Can you work these out from the model? Positions are in its coordinate system, mm. A direction names the side the tool comes from. Give positions to 0.01 mm unless a question says otherwise; leave off trailing zeros. Order: outer loops, then holes, each group sorted by start corner. A loop starts at its lowest first (then second) coordinate and runs counter-clockwise, first axis right, second up. Notation, with made-up numbers: M -7,11.5 L 2,11.5 A22 cw 2,23.5 Z; hole C 13,22 d1. An arc over 180 degrees is marked long. Answer as a JSON object with one key per item and string values.
```python
from build123d import *

# Parameters (mm, degrees)
EXTRUDE_1_DEPTH     = 10
SKETCH_2_R          = 10
CUT_EXTRUDE_1_DEPTH = 62.846584384
SKETCH_3_R          = 20
SKETCH_3_R_2        = 15
EXTRUDE_2_DEPTH     = 35
EXTRUDE_3_DEPTH     = 10
EXTRUDE_4_REACH     = 119.473
CUT_EXTRUDE_3_DEPTH = 10
EXTRUDE_5_DEPTH     = 10


with BuildPart() as part:
    # Sketch 1 → Extrude 1 (new body)
    with BuildSketch(Plane.XY):
        with BuildLine():
            Line((50, 35), (-50, 35))
            Line((-50, 35), (-50, -15))
            ThreePointArc((-50, -15), (-44.142135624, -29.142135624), (-30, -35))
            Line((-30, -35), (30, -35))
            ThreePointArc((30, -35), (44.142135624, -29.142135624), (50, -15))
            Line((50, -15), (50, 35))
        make_face()
    extrude(amount=-EXTRUDE_1_DEPTH)

    # Sketch 2 → Cut-Extrude 1 (cut, through all)
    with BuildSketch(Plane(origin=(0, 0, -10), x_dir=(-1, 0, 0), z_dir=(0, 0, -1))):
        with Locations((-30, -15)):
            Circle(SKETCH_2_R)
        with Locations((30, -15)):
            Circle(SKETCH_2_R)
    extrude(amount=-CUT_EXTRUDE_1_DEPTH, mode=Mode.SUBTRACT)



with BuildPart() as body_2:
    # Sketch 3 → Extrude 2 (new body)
    with BuildSketch(Plane(origin=(0, 35, 0), x_dir=(1, 0, 0), z_dir=(0, 1, 0))):
        with Locations(Location((0, 60, 0), (0, 0, 180))):
            Circle(SKETCH_3_R)
        with Locations(Location((0, 60, 0), (0, 0, 180))):
            Circle(SKETCH_3_R_2, mode=Mode.SUBTRACT)
    extrude(amount=-EXTRUDE_2_DEPTH)


with BuildPart() as part_1:
    add(part.part)

    add(body_2.part)  # Extrude 3 merges body 2
    # Sketch 4 → Extrude 3 (add)
    with BuildSketch(Plane(origin=(0, 35, 0), x_dir=(1, 0, 0), z_dir=(0, 1, 0))):
        with BuildLine():
            Line((-20, 60), (-50, 10))
            Line((-50, 10), (50, 10))
            Line((50, 10), (20, 60))
            ThreePointArc((20, 60), (0, 40), (-20, 60))
        make_face()
    extrude(amount=-EXTRUDE_3_DEPTH)

    # Extrude 4: up to this face of the body (flat: up to its plane)
    extrude_4_end = Plane(part_1.part.faces().sort_by_distance((0, 25, -27.034412528))[0])
    # Sketch 6 → Extrude 4 (add, up to the picked face)
    with BuildSketch(Plane.XZ.offset(35), mode=Mode.PRIVATE) as extrude_4_sk1:
        with BuildLine():
            Line((5, -40.635083269), (5, -10))
            Line((5, -10), (0, -10))
            Line((0, -10), (-5, -10))
            Line((-5, -10), (-5, -40.635083269))
            ThreePointArc((-5, -40.635083269), (0, -40), (5, -40.635083269))
        make_face()
    extrude_4_tool1 = split(extrude(extrude_4_sk1.sketch, amount=-EXTRUDE_4_REACH, mode=Mode.PRIVATE), bisect_by=extrude_4_end, keep=Keep.BOTH, mode=Mode.PRIVATE)
    add(extrude_4_tool1.solids().sort_by(Axis((0, -35, -25.105756), (0, 1, 0)))[0])

    # Sketch 7 → Cut-Extrude 3 (cut)
    with BuildSketch(Plane.ZY.offset(5)):
        Polygon((-10, -35), (-40.635083269, 0), (-40.635083269, -35), align=None)
    extrude(amount=-CUT_EXTRUDE_3_DEPTH, mode=Mode.SUBTRACT)

    # Sketch 8 → Extrude 5 (add)
    # profile 1 of 2: a face of its own
    with BuildSketch(Plane.XY.offset(-85)):
        with BuildLine():
            ThreePointArc((10, 10), (-7.071067812, 17.071067812), (0, 0))
            ThreePointArc((0, 0), (7.071067812, 2.928932188), (10, 10))
        make_face()
        with BuildLine():
            ThreePointArc((7, 10), (4.949747468, 5.050252532), (0, 3))
            ThreePointArc((0, 3), (-4.949747468, 14.949747468), (7, 10))
        make_face(mode=Mode.SUBTRACT)
    # profile 2 of 2: a face of its own
    with BuildSketch(Plane.XY.offset(-85)):
        with BuildLine():
            ThreePointArc((10, 10), (-7.071067812, 17.071067812), (0, 0))
            ThreePointArc((0, 0), (7.071067812, 2.928932188), (10, 10))
        make_face()
        with BuildLine():
            ThreePointArc((7, 10), (4.949747468, 5.050252532), (0, 3))
            ThreePointArc((0, 3), (-4.949747468, 14.949747468), (7, 10))
        make_face(mode=Mode.SUBTRACT)
    extrude(amount=EXTRUDE_5_DEPTH)


solid = part_1.part
```
1) I want a section at C-C on x = -2.5. Write out the boundary of the cut face in (y, z), and give its area (3 significant figures).
Results found:
{"outline": "M -35,-10 L -0.55,-40.16 L 0,-40.16 L 0,-45.21 L 35,-45.21 L 35,0 L -35,0 Z; M 0,-79.84 L 0.32,-79.84 L 0.32,-85 L 3.46,-85 L 3.46,-79.84 L 16.54,-79.84 L 16.54,-85 L 19.68,-85 L 19.68,-79.84 L 35,-79.84 L 35,-74.79 L 0,-74.79 Z", "area": "2,680 mm²"}
2) I want a section at A-A on z = -56. Write out the boundary of the cut face in (x, y).
Results found:
{"outline": "M -22.4,25 L -19.6,25 L -19.6,0 L -14.46,0 L -14.46,35 L -22.4,35 Z; M 14.46,0 L 19.6,0 L 19.6,25 L 22.4,25 L 22.4,35 L 14.46,35 Z"}
3) I need wall thicknesses on L1, parallel to Z at x = 0, y = 22; L2, parallel to Y at x = 30, z = -4.5; L3, parallel to Z at x = -8, y = 11.5. Which ranges of each line are inside material? Lowest first, please.
Results found:
{"L1": "z = -80 to -75, -45 to 0", "L2": "y = -35 to -25, -5 to 35", "L3": "z = -85 to -72.69, -47.31 to -41.67, -10 to 0"}
4) I want a section at B-B on y = -18.5. Write out the boundary of the cut face in (x, z), and give its area (3 significant figures).
Results found:
{"outline": "M -49.69,-10 L -39.37,-10 L -39.37,0 L -49.69,0 Z; M -20.63,-10 L -5,-10 L -5,-24.44 L 5,-24.44 L 5,-10 L 20.63,-10 L 20.63,0 L -20.63,0 Z; M 39.37,-10 L 49.69,-10 L 49.69,0 L 39.37,0 Z", "area": "764 mm²"}
5) I'm going to push flat-ended pins straight in: pin 1 Ø22.5 at (x, y) = (0, 10) entering from -Z; pin 2 Ø8 at (x, z) = (-17, -32) entering from -Y; pin 3 Ø22.5 at (x, z) = (18, -41.5) entering from -Y; pin 4 Ø13.5 at (x, y) = (34.5, -20) entering from -Z. Where does each tip first touch, or does it pass through?
Results found:
{"pin 1": "stops at z = -85", "pin 2": "stops at y = 25", "pin 3": "stops at y = 0", "pin 4": "stops at z = -10"}
6) For faces 4 (the face through (-44.297, -28.986, -4.93)), 5 (the face through (22, 25, -30)), 6 (the face through (-23, 25, -30)), which set-ups out of +Z, -Z, +X, -X, +Y, -Y let a thin tool reach every point of the face, with its end or its side?
Results found:
{"face 4": "+Z, -Z, -X, -Y", "face 5": "+X, -Y", "face 6": "-X, -Y"}
7) Thinking about a two-plate mould opening in Y: for faces 1 (the face through (5, 1, -22)), 2 (the face through (-39.54, -12, -5.07)), 3 (the face through (0, -35, -5)), which applies, pulls with the +Y half, pulls with the -Y half, needs draft (parallel to the pull), parting line crosses it, or undercut?
Results found:
{"face 1": "needs draft", "face 2": "undercut", "face 3": "pulls with the -Y half"}
8) I want a section at D-D on z = -72. Write out the boundary of the cut face in (x, y).
Results found:
{"outline": "M -16,0 L -9,0 L -9,35 L -16,35 Z; M 9,0 L 16,0 L 16,35 L 9,35 Z"}
